CAD build for the part. Positions are in the model's coordinates, mm. A direction names the side the tool comes from. Give positions to 0.01 mm unless a question says otherwise; leave off trailing zeros. Write each loop counter-clockwise with the first axis right and the second up, starting at its lowest first coordinate (ties: lowest second). Pieces come first, ordered by that corner, then holes. Notation, with made-up numbers: M 89,4 L 94,4 A28 ccw 94,34 Z; hole C -39,76 d6. An arc over 180 degrees is marked long. One line per question, with ' | ' between items. Start each with the question number.
1. Pull direction Z, two halves, no side cores. Call faces 5 (the face through (-12.74, 8.51, -14.15)), 6 (the face through (-7, 9.2, -10.85)), 7 (the face through (-9.8, 0.88, -7.42)): released by +Z, released by -Z, zero draft, split by the parting line, or undercut.
2. Cut at A-A, the plane y = 3. Write the cut outline in (x, z), then the cut area to 3 significant figures.
3. Wall check: L1, parallel to Z at x = 10, y = 5.25; L2, parallel to X at y = 4.75, z = 7.5. Give the ranges that are in metal, low to high.
4. Cut at C-C, the plane x = -4. Write the cut outline in (y, z).
5. Which spindle directions (+Z, -Z, +X, -X, +Y, -Y) get a long thin tool onto all of the face, cutting with end or side? Do faces 1 (the face through (-6.19, 9.54, 0.15)), 2 (the face through (-12.74, 8.51, 14.05)), 3 (the face through (-8.75, 5.69, 7.45)), 4 (the face through (0, 9, -14)). Say none if no direction does.
6. Flat gauge pins, fed straight in: pin 1 (5.5 mm diameter, centred on x = 1, z = 3.5, fed in from -Y); pin 2 (3 mm diameter, centred on x = 4.5, y = 2, fed in from +Z); pin 3 (2 mm diameter, centred on y = 5.5, z = 14.5, fed in from -X); pin 4 (10 mm diameter, centred on x = -1, z = 2.5, fed in from +Y). Where does each tip first touch, or does it go through?
7. Cut at D-D, the plane y = 5.5. Write the cut outline in (x, z).
8. Cut at B-B, the plane z = -12. Write the cut outline in (x, y), then the cut area to 3 significant figures.
```python
from build123d import *

# Parameters (mm, degrees)
MAINBLOCKSKETCH_W              = 26.5
MAINBLOCKSKETCH_H              = 34.7
MAINBLOCK_DEPTH                = 9
FACEDSURFACESKETCH_W           = 27
FACEDSURFACESKETCH_H           = 21.7
FACEDSURFACE_DEPTH             = 10
M3X0_5_TAPPED_HOLE1_D          = 2.5
M3X0_5_TAPPED_HOLE1_DEPTH      = 8.5
M3X0_5_TAPPED_HOLE1_TIP        = 0.751075774
RAIL_SLOT_DEPTH                = 25.151035175
RAIL_SLOT_DEPTH_BACK           = 25.151035175
INTERNAL_DIP_SKETCH_W          = 13.5
INTERNAL_DIP_SKETCH_H          = 21.7
INTERNAL_DIP_DEPTH             = 0.9
INTERNAL_CHAMFER_SIZE          = 0.5
COSMETIC_CHAMFERS_SIZE         = 1
SMALLER_COSMETIC_CHAMFERS_SIZE = 0.5


with BuildPart() as part:
    # MainBlockSketch → MainBlock (new body)
    with BuildSketch(Plane(origin=(0, 0, 0), x_dir=(1, 0, 0), z_dir=(0, 1, 0))):
        Rectangle(MAINBLOCKSKETCH_W, MAINBLOCKSKETCH_H)
    extrude(amount=MAINBLOCK_DEPTH)

    # FacedSurfaceSketch → FacedSurface (add)
    with BuildSketch(Plane(origin=(0, 0, 0), x_dir=(1, 0, 0), z_dir=(0, 1, 0))):
        Rectangle(FACEDSURFACESKETCH_W, FACEDSURFACESKETCH_H)
    extrude(amount=FACEDSURFACE_DEPTH)

    # M3x0.5 Tapped Hole1
    with Locations(Plane(origin=(0, 10, 0), x_dir=(1, 0, 0), z_dir=(0, 1, 0))):
        with Locations((-10, 7.5), (10, 7.5), (10, -7.5), (-10, -7.5)):
            Hole(M3X0_5_TAPPED_HOLE1_D / 2, depth=M3X0_5_TAPPED_HOLE1_DEPTH)
            with Locations((0, 0, -(M3X0_5_TAPPED_HOLE1_DEPTH + M3X0_5_TAPPED_HOLE1_TIP / 2))):  # 118° drill point
                Cone(0, M3X0_5_TAPPED_HOLE1_D / 2, M3X0_5_TAPPED_HOLE1_TIP, mode=Mode.SUBTRACT)

    # RailSlotSketch → Rail Slot (cut, two sides: drawn at the far end of the back side and taken through both)
    with BuildSketch(Plane.XY.offset(-RAIL_SLOT_DEPTH_BACK)):
        with BuildLine():
            Line((-6, 2.59), (-6, 5))
            Line((-6, 5), (6, 5))
            Line((6, 5), (6, 2.59))
            ThreePointArc((6, 2.59), (5.2, 1.79), (6, 0.99))
            Line((6, 0.99), (6, 0))
            Line((6, 0), (-6, 0))
            Line((-6, 0), (-6, 0.99))
            ThreePointArc((-6, 0.99), (-5.2, 1.79), (-6, 2.59))
        make_face()
    extrude(amount=RAIL_SLOT_DEPTH + RAIL_SLOT_DEPTH_BACK, mode=Mode.SUBTRACT)

    # Internal Dip Sketch → Internal Dip (cut)
    with BuildSketch(Plane(origin=(0, 10, 0), x_dir=(1, 0, 0), z_dir=(0, 1, 0))):
        Rectangle(INTERNAL_DIP_SKETCH_W, INTERNAL_DIP_SKETCH_H)
    extrude(amount=-INTERNAL_DIP_DEPTH, mode=Mode.SUBTRACT)

    # Internal Chamfer
    internal_chamfer_edges = [part.edges().sort_by_distance(p)[0] for p in [
        (6, 5, 0),
        (-6, 5, 0),
    ]]
    chamfer(internal_chamfer_edges, length=INTERNAL_CHAMFER_SIZE)

    # Cosmetic Chamfers
    # the kernel refuses this chamfer: 1 mm, written as the material it adds along each edge
    with BuildSketch(Plane(origin=(-6.75, 9.1, 10.85), x_dir=(0.9996219169112968, -0.027495876610585623, 0), z_dir=(0, 0, -1))) as cosmetic_chamfers_piece_1_section:
        Polygon((COSMETIC_CHAMFERS_SIZE * 0.999621916911, -COSMETIC_CHAMFERS_SIZE * 0.0274958766106), (-COSMETIC_CHAMFERS_SIZE * 0.0274958766106, -COSMETIC_CHAMFERS_SIZE * 0.999621916911), (0, 0), align=None)
    cosmetic_chamfers_piece_1 = extrude(amount=21.7, mode=Mode.PRIVATE)
    cosmetic_chamfers_piece_1 = split(cosmetic_chamfers_piece_1, bisect_by=Plane(origin=(-6.414099253, 10, 0), z_dir=(0, -1, 0)), keep=Keep.TOP, mode=Mode.PRIVATE)
    add(cosmetic_chamfers_piece_1)
    with BuildSketch(Plane(origin=(6.75, 9.1, -10.85), x_dir=(0.02749587661058651, 0.9996219169112968, 0), z_dir=(0, 0, 1))) as cosmetic_chamfers_piece_2_section:
        Polygon((COSMETIC_CHAMFERS_SIZE * 0.999621916911, COSMETIC_CHAMFERS_SIZE * 0.0274958766106), (-COSMETIC_CHAMFERS_SIZE * 0.0274958766106, COSMETIC_CHAMFERS_SIZE * 0.999621916911), (0, 0), align=None)
    cosmetic_chamfers_piece_2 = extrude(amount=21.7, mode=Mode.PRIVATE)
    cosmetic_chamfers_piece_2 = split(cosmetic_chamfers_piece_2, bisect_by=Plane(origin=(6.414099253, 10, 0), z_dir=(0, -1, 0)), keep=Keep.TOP, mode=Mode.PRIVATE)
    add(cosmetic_chamfers_piece_2)
    # the kernel refuses this chamfer: 1 mm, written as the material it takes off along each edge
    with BuildSketch(Plane(origin=(13.25, 9, 19.921682988), x_dir=(0.027495876610585623, -0.9996219169112968, 0), z_dir=(0, 0, -1))) as cosmetic_chamfers_2_piece_1:
        Polygon((COSMETIC_CHAMFERS_SIZE * 0.999621916911, COSMETIC_CHAMFERS_SIZE * 0.0274958766106), (-COSMETIC_CHAMFERS_SIZE * 0.0274958766106, COSMETIC_CHAMFERS_SIZE * 0.999621916911), (0, 0), align=None)
    extrude(amount=9.071682988, mode=Mode.SUBTRACT)
    with BuildSketch(Plane(origin=(-13.25, 9, 10.85), x_dir=(0.9996219169112968, 0.027495876610585647, 0), z_dir=(0, 0, 1)), Plane(origin=(-13.25, 9, -19.921682988), x_dir=(0.9996219169112968, 0.027495876610585647, 0), z_dir=(0, 0, 1)), Plane(origin=(13.25, 9, -10.85), x_dir=(-0.9996219169112968, 0.027495876610585647, 0), z_dir=(0, 0, -1))) as cosmetic_chamfers_2_piece_2:
        Polygon((COSMETIC_CHAMFERS_SIZE * 0.999621916911, -COSMETIC_CHAMFERS_SIZE * 0.0274958766106), (-COSMETIC_CHAMFERS_SIZE * 0.0274958766106, -COSMETIC_CHAMFERS_SIZE * 0.999621916911), (0, 0), align=None)
    extrude(amount=9.071682988, mode=Mode.SUBTRACT)

    # Smaller Cosmetic Chamfers
    smaller_cosmetic_chamfers_edges = [part.edges().sort_by_distance(p)[0] for p in [
        (13.5, 10, 0),
        (-13.5, 10, 0),
        (-13.5, 0, 0),
        (13.5, 0, 0),
        (6, 0, 0),
        (-6, 0, 0),
    ]]
    chamfer(smaller_cosmetic_chamfers_edges, length=SMALLER_COSMETIC_CHAMFERS_SIZE)


solid = part.part
```
Here are the results:
1) face 5: zero draft | face 6: released by -Z | face 7: undercut
2) outline: M -13.5,-10.85 L -13.25,-10.85 L -13.25,-17.35 L -6,-17.35 L -6,17.35 L -13.25,17.35 L -13.25,10.85 L -13.5,10.85 Z; M 6,-17.35 L 13.25,-17.35 L 13.25,-10.85 L 13.5,-10.85 L 13.5,10.85 L 13.25,10.85 L 13.25,17.35 L 6,17.35 Z; hole C -10,-7.5 d2.5; hole C -10,7.5 d2.5; hole C 10,-7.5 d2.5; hole C 10,7.5 d2.5 | area: 494 mm^2
3) L1: -17.35 to -8.75, -6.25 to 6.25, 8.75 to 17.35 | L2: -13.5 to -11.25, -8.75 to -5.75, 5.75 to 8.75, 11.25 to 13.5
4) outline: M 5,-17.35 L 9,-17.35 L 9,-10.85 L 9.1,-10.85 L 9.1,10.85 L 9,10.85 L 9,17.35 L 5,17.35 Z
5) face 1: +Z, -Z, +Y | face 2: +Z, -X, +Y | face 3: +Y | face 4: -Z, +X, -X, +Y
6) pin 1: y = 5 | pin 2: z = 17.35 | pin 3: x = -13.25 | pin 4: y = 9.35
7) outline: M -13.5,-10.85 L -13.25,-10.85 L -13.25,-17.35 L 13.25,-17.35 L 13.25,-10.85 L 13.5,-10.85 L 13.5,10.85 L 13.25,10.85 L 13.25,17.35 L -13.25,17.35 L -13.25,10.85 L -13.5,10.85 Z; hole C -10,-7.5 d2.5; hole C -10,7.5 d2.5; hole C 10,-7.5 d2.5; hole C 10,7.5 d2.5
8) outline: M -13.25,0.25 L -13,0 L -6.5,0 L -6,0.5 L -6,0.99 A0.8 ccw -6,2.59 L -6,4.5 L -5.5,5 L 5.5,5 L 6,4.5 L 6,2.59 A0.8 ccw 6,0.99 L 6,0.5 L 6.5,0 L 13,0 L 13.25,0.25 L 13.25,8 L 12.25,9 L -12.25,9 L -13.25,8 Z | area: 179 mm^2
